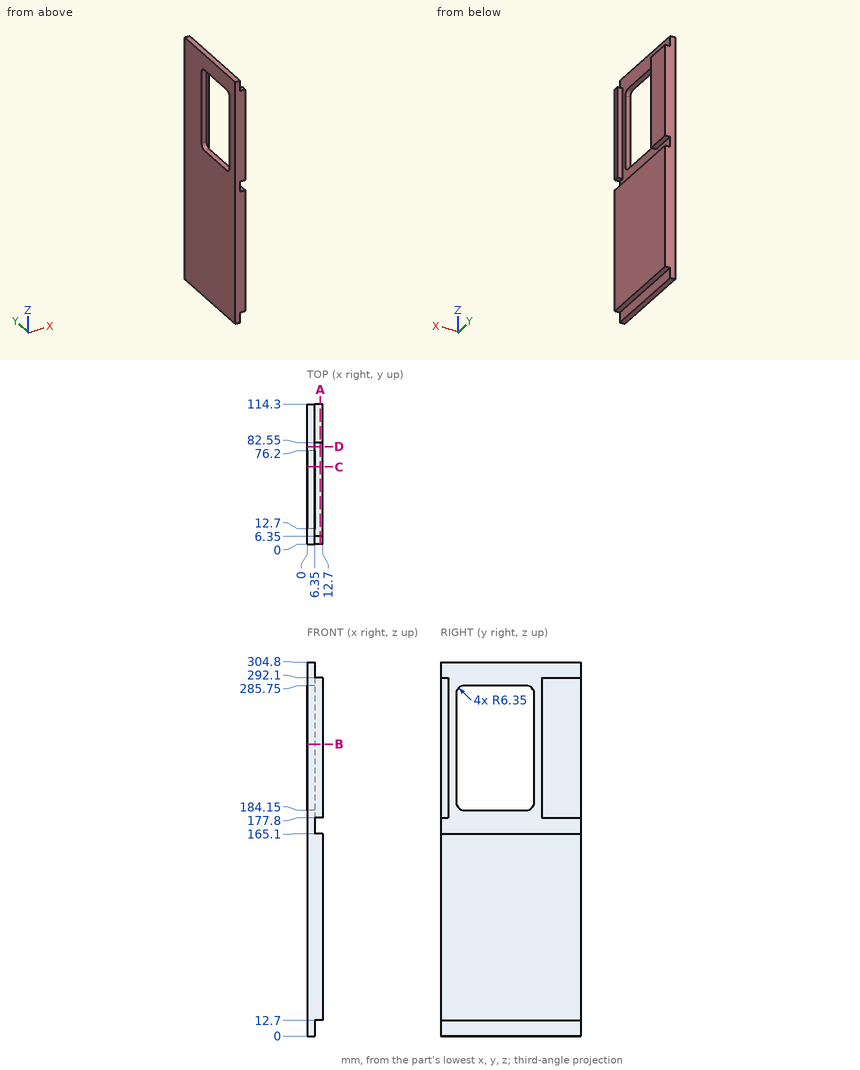
For this review, use the dimensioned drawing (mm, ordinates from the lowest corner) and the shaded views. Coordinates: 2 decimals unless noted, no trailing zeros. Loops run counter-clockwise (first coordinate to the right, second up) from the corner with the lowest first, then second, coordinate; pieces in that order, holes last. Notation, with made-up numbers: (-34.5, -9.75) -> (-5.5, -9.75) arc R26 ccw to (-5.5, 29.25) -> close; hole circle Ø1 at (62, 37.25). An arc over 180 degrees is marked (long way). Return JSON: item names as keys, results as strings. Group by question number.
(1) Consider section C-C, the plane y = 63. Give the boundary of the cut face in (x, z), plus the area to 3 significant figures.
(2) Consider section B-B, the plane z = 238. Give the boundary of the cut face in (x, y), plus the area to 3 significant figures.
(3) Consider section D-D, the plane y = 79.5. Give the boundary of the cut face in (x, z), plus the area to 3 significant figures.
(4) Consider section A-A, the plane x = 10.75. Give the boundary of the cut face in (y, z), plus the area to 3 significant figures.
(5) To check wall thickness, follow L1, parallel to Z at x = 6, y = 25.5; L2, parallel to Y at x = 2, z = 218.5; L3, parallel to Y at x = 8.5, z = 243. State the ranges of each line that lie inside material, in increasing order.
(6) For pin 1 Ø3 at (x, y) = (10, 3) entering from -Z; pin 2 Ø5 at (x, y) = (9.5, 3.5) entering from +Z; pin 3 Ø6.5 at (y, z) = (45, 5) entering from +X, all flat-tipped, find the tip position at first contact; note any pin that passes through.
Results below:
{
 "1": {"outline": "(0, 0) -> (6.35, 0) -> (6.35, 12.7) -> (12.7, 12.7) -> (12.7, 165.1) -> (6.35, 165.1) -> (6.35, 184.15) -> (0, 184.15) -> close; (0, 285.75) -> (6.35, 285.75) -> (6.35, 304.8) -> (0, 304.8) -> close", "area": "2,260 mm2"},
 "2": {"outline": "(0, 0) -> (12.7, 0) -> (12.7, 6.35) -> (6.35, 6.35) -> (6.35, 12.7) -> (0, 12.7) -> close; (0, 76.2) -> (6.35, 76.2) -> (6.35, 82.55) -> (12.7, 82.55) -> (12.7, 114.3) -> (0, 114.3) -> close", "area": "565 mm2"},
 "3": {"outline": "(0, 0) -> (6.35, 0) -> (6.35, 12.7) -> (12.7, 12.7) -> (12.7, 165.1) -> (6.35, 165.1) -> (6.35, 304.8) -> (0, 304.8) -> close", "area": "2,900 mm2"},
 "4": {"outline": "(0, 12.7) -> (114.3, 12.7) -> (114.3, 165.1) -> (0, 165.1) -> close; (0, 177.8) -> (6.35, 177.8) -> (6.35, 292.1) -> (0, 292.1) -> close; (82.55, 177.8) -> (114.3, 177.8) -> (114.3, 292.1) -> (82.55, 292.1) -> close", "area": "21,800 mm2"},
 "5": {"L1": "z = 0 to 184.15, 285.75 to 304.8", "L2": "y = 0 to 12.7, 76.2 to 114.3", "L3": "y = 0 to 6.35, 82.55 to 114.3"},
 "6": {"pin 1": "stops at z = 12.7", "pin 2": "stops at z = 292.1", "pin 3": "stops at x = 6.35"}
}
